Geometry check sheet. Reference: the model listing, model coordinates, mm. A direction names the side the tool comes from. Coordinates: 2 decimals unless noted, no trailing zeros. Write each loop counter-clockwise with the first axis right and the second up, starting at its lowest first coordinate (ties: lowest second). Pieces come first, ordered by that corner, then holes. Notation, with made-up numbers: (67.5, 79) - (107.5, 79) arc R14 cw to (107.5, 96) - close; hole circle Ø2 at (15.25, -12.75). An arc over 180 degrees is marked (long way). Answer as a JSON object with one key per item and string values. Group by question number.
from build123d import *

# Parameters (mm, degrees)
SKETCH1_W           = 45
SKETCH1_H           = 47
BOSS_EXTRUDE1_DEPTH = 2
SKETCH2_W           = 45
SKETCH2_H           = 2
BOSS_EXTRUDE2_DEPTH = 19.5
FILLET1_R           = 2
FILLET2_R           = 5
SKETCH3_W           = 25
SKETCH3_H           = 22.5
CUT_EXTRUDE1_DEPTH  = 39.99679474
SKETCH4_R           = 1.5
CUT_EXTRUDE2_DEPTH  = 54.958317246
SKETCH5_W           = 25
SKETCH5_H           = 22.5
CUT_EXTRUDE3_DEPTH  = 10


with BuildPart() as part:
    # Sketch1 → Boss-Extrude1 (new body)
    with BuildSketch(Plane.XY):
        Rectangle(SKETCH1_W, SKETCH1_H)
    extrude(amount=BOSS_EXTRUDE1_DEPTH)

    # Sketch2 → Boss-Extrude2 (add)
    with BuildSketch(Plane(origin=(0, 0, 0), x_dir=(-1, 0, 0), z_dir=(0, 0, -1))):
        with Locations((0, -22.5)):
            Rectangle(SKETCH2_W, SKETCH2_H)
    extrude(amount=BOSS_EXTRUDE2_DEPTH)

    # Fillet1
    fillet1_edges = [part.edges().sort_by_distance(p)[0] for p in [
        (0, -23.5, 2),
    ]]
    fillet(fillet1_edges, radius=FILLET1_R)

    # Fillet2
    fillet2_edges = [part.edges().sort_by_distance(p)[0] for p in [
        (22.5, -22.5, -19.5),
        (-22.5, -22.5, -19.5),
    ]]
    fillet(fillet2_edges, radius=FILLET2_R)

    # Sketch3 → Cut-Extrude1 (cut, through all)
    with BuildSketch(Plane.XY.offset(2)):
        with Locations((0, 12.25)):
            Rectangle(SKETCH3_W, SKETCH3_H)
    extrude(amount=-CUT_EXTRUDE1_DEPTH, mode=Mode.SUBTRACT)

    # Sketch4 → Cut-Extrude2 (cut, through all)
    with BuildSketch(Plane(origin=(0, -21.5, 0), x_dir=(1, 0, 0), z_dir=(0, 1, 0))):
        with Locations(Location((0, 14.5, 0), (0, 0, 180))):
            Circle(SKETCH4_R)
    extrude(amount=-CUT_EXTRUDE2_DEPTH, mode=Mode.SUBTRACT)

    # Sketch5 → Cut-Extrude3 (cut)
    with BuildSketch(Plane(origin=(0, 0, 0), x_dir=(-1, 0, 0), z_dir=(0, 0, -1))):
        with Locations((0, -10.25)):
            Rectangle(SKETCH5_W, SKETCH5_H)
    extrude(amount=-CUT_EXTRUDE3_DEPTH, mode=Mode.SUBTRACT)


solid = part.part
(1) Material ranges on L1, parallel to Y at x = 13, z = -8.75; L2, parallel to Z at x = 20, y = -15; L3, parallel to Z at x = 0, y = -22, recorded low to high. Write a range as [from, to].
(2) Section check B-B (y = -6). Record the cut outline in (x, z).
(3) Gauge pin test, flat ends, axial feed: pin 1 (3 mm diameter, centred on x = 13.5, y = -18.5, fed in from -Z); pin 2 (1.5 mm diameter, centred on x = -17.5, z = -1, fed in from +Y). Record the tip position at first contact, or that the pin passes through.
(4) Draft check along X on faces 1 (the face through (21.07, -22.49, -18)), 2 (the face through (12.5, 1, 1)), 3 (the face through (-22.5, -5, 1)), 4 (the face through (0.32, -22.93, 1.4)). Enter one of: +X half, -X half, draft (parallel to the pull), parting line (faces both ways), or undercut.
(5) Section check D-D (x = -8). Record the cut outline in (y, z).
(6) Section check A-A (x = 0). Record the cut outline in (y, z).
(7) Section check C-C (z = 0.75). Record the cut outline in (x, y), and give its area (3 significant figures).
(8) Set-up check for faces 5 (the face through (-12.5, 1, 1)), 6 (the face through (0, -22, -19.5)), 7 (the face through (17, 1, 0)): record each of +Z, -Z, +X, -X, +Y, -Y from which the full face is reachable in a straight line by a thin tool's end or side.
Conclusion:
{
 "1": {"L1": "y = [-23.5, -21.5]", "L2": "z = [0, 2]", "L3": "z = [-19.5, -16], [-13, 1.94]"},
 "2": {"outline": "(-22.5, 0) - (-12.5, 0) - (-12.5, 2) - (-22.5, 2) - close; (12.5, 0) - (22.5, 0) - (22.5, 2) - (12.5, 2) - close"},
 "3": {"pin 1": "stops at z = 0", "pin 2": "stops at y = -21.5"},
 "4": {"face 1": "+X half", "face 2": "undercut", "face 3": "-X half", "face 4": "draft"},
 "5": {"outline": "(-23.5, -19.5) - (-21.5, -19.5) - (-21.5, 2) arc R2 ccw to (-23.5, 0) - close"},
 "6": {"outline": "(-23.5, -19.5) - (-21.5, -19.5) - (-21.5, -16) - (-23.5, -16) - close; (-23.5, -13) - (-21.5, -13) - (-21.5, 2) arc R2 ccw to (-23.5, 0) - close"},
 "7": {"outline": "(-22.5, -23.35) - (22.5, -23.35) - (22.5, 23.5) - (12.5, 23.5) - (12.5, -21.5) - (-12.5, -21.5) - (-12.5, 23.5) - (-22.5, 23.5) - close", "area": "983 mm^2"},
 "8": {"face 5": "+Z, -Z, +Y", "face 6": "-Z, +X, -X, +Y, -Y", "face 7": "-Z, +X, -X, +Y"}
}
